from build123d import *

# Parameters (mm, degrees)
SKETCH1_W            = 1017.150431592
SKETCH1_H            = 1007.380411388
BOSS_EXTRUDE1_DEPTH  = 10
SKETCH2_W            = 622.325209365
SKETCH2_H            = 576.276335175
SKETCH2_W_2          = 550.905616221
SKETCH2_H_2          = 495.653174758
BOSS_EXTRUDE2_DEPTH  = 700
BOSS_EXTRUDE3_DEPTH  = 10
SKETCH4_W            = 343.745663019
SKETCH4_H            = 631.457492732
CUT_EXTRUDE1_DEPTH   = 40
SKETCH5_W            = 96.085656893
SKETCH5_H            = 209.087602639
BOSS_EXTRUDE4_DEPTH  = 1
SKETCH6_W            = 75.527574186
SKETCH6_H            = 43.688329808
CUT_EXTRUDE2_DEPTH   = 1
SKETCH7_R            = 20.29708438
SKETCH7_R_2          = 20.231985555
BOSS_EXTRUDE5_DEPTH  = 1
BOSS_EXTRUDE6_DEPTH  = 1
SKETCH9_W            = 27.290112983
SKETCH9_H            = 631.457492732
BOSS_EXTRUDE7_DEPTH  = 170
SKETCH10_W           = 23.826275683
SKETCH10_H           = 630.503372623
BOSS_EXTRUDE8_DEPTH  = 170
SKETCH11_W           = 102.432085561
SKETCH11_H           = 42.683052162
BOSS_EXTRUDE9_DEPTH  = 1
SKETCH12_W           = 89.43349782
SKETCH12_H           = 33.905937228
CUT_EXTRUDE3_DEPTH   = 1
BOSS_EXTRUDE10_DEPTH = 1
BOSS_EXTRUDE11_DEPTH = 1
BOSS_EXTRUDE12_DEPTH = 1
SKETCH16_W           = 75.527574186
SKETCH16_H           = 43.688329808
CUT_EXTRUDE4_DEPTH   = 2
CUT_EXTRUDE5_DEPTH   = 1
SKETCH18_W           = 75.494640665
SKETCH18_H           = 38.009856791
CUT_EXTRUDE6_DEPTH   = 3
BOSS_EXTRUDE14_DEPTH = 2
BOSS_EXTRUDE15_DEPTH = 2


with BuildPart() as part:
    # Sketch1 → Boss-Extrude1 (new body)
    with BuildSketch(Plane(origin=(0, 0, 0), x_dir=(1, 0, 0), z_dir=(0, 1, 0))):
        Rectangle(SKETCH1_W, SKETCH1_H)
    extrude(amount=BOSS_EXTRUDE1_DEPTH)

    # Sketch2 → Boss-Extrude2 (add)
    with BuildSketch(Plane(origin=(0, 10, 0), x_dir=(1, 0, 0), z_dir=(0, 1, 0))):
        with Locations((0.175057265, -25.815388539)):
            Rectangle(SKETCH2_W, SKETCH2_H)
        with Locations((3.438260109, -29.815460152)):
            Rectangle(SKETCH2_W_2, SKETCH2_H_2, mode=Mode.SUBTRACT)
    extrude(amount=BOSS_EXTRUDE2_DEPTH)

    # Sketch3 → Boss-Extrude3 (add)
    with BuildSketch(Plane(origin=(0, 710, 0), x_dir=(1, 0, 0), z_dir=(0, 1, 0))):
        Polygon((-310.987547417, 262.322779049), (311.337661948, 262.322779049), (311.337661948, -314.105065769), (-310.987547417, -313.953556126), align=None)
    extrude(amount=BOSS_EXTRUDE3_DEPTH)

    # Sketch4 → Cut-Extrude1 (cut)
    with BuildSketch(Plane.XY.offset(313.953556126)):
        with Locations((1.971257292, 325.728746366)):
            Rectangle(SKETCH4_W, SKETCH4_H)
    extrude(amount=-CUT_EXTRUDE1_DEPTH, mode=Mode.SUBTRACT)

    # Sketch5 → Boss-Extrude4 (add)
    with BuildSketch(Plane.XY.offset(313.953556126)):
        with Locations((-235.628465158, 369.989290471)):
            Rectangle(SKETCH5_W, SKETCH5_H)
    extrude(amount=BOSS_EXTRUDE4_DEPTH)

    # Sketch6 → Cut-Extrude2 (cut)
    with BuildSketch(Plane.XY.offset(314.953556126)):
        with Locations((-233.410831007, 396.905866965)):
            Rectangle(SKETCH6_W, SKETCH6_H)
    extrude(amount=-CUT_EXTRUDE2_DEPTH, mode=Mode.SUBTRACT)

    # Sketch7 → Boss-Extrude5 (add)
    with BuildSketch(Plane.XY.offset(314.953556126)):
        with Locations((-236.075713016, 343.617219623)):
            Circle(SKETCH7_R)
        with Locations((-236.075713016, 291.501520139)):
            Circle(SKETCH7_R_2)
    extrude(amount=BOSS_EXTRUDE5_DEPTH)

    # Sketch8 → Boss-Extrude6 (add)
    with BuildSketch(Plane.XY.offset(315.953556126)):
        Polygon((-248.100542069, 334.343180385), (-224.116847865, 334.343180385), (-236.108694967, 356.570085863), align=None)
        Polygon((-248.100542069, 300.734143469), (-224.116847865, 300.734143469), (-236.108694967, 278.021129489), align=None)
    extrude(amount=BOSS_EXTRUDE6_DEPTH)

    # Sketch9 → Boss-Extrude7 (add)
    with BuildSketch(Plane(origin=(-169.901574217, 0, 0), x_dir=(0, 0, -1), z_dir=(1, 0, 0))):
        with Locations((-291.287104022, 325.728746366)):
            Rectangle(SKETCH9_W, SKETCH9_H)
    extrude(amount=BOSS_EXTRUDE7_DEPTH)

    # Sketch10 → Boss-Extrude8 (add)
    with BuildSketch(Plane(origin=(0.098425783, 0, 0), x_dir=(0, 0, -1), z_dir=(1, 0, 0))):
        with Locations((-289.555185372, 325.251686312)):
            Rectangle(SKETCH10_W, SKETCH10_H)
    extrude(amount=BOSS_EXTRUDE8_DEPTH)

    # Sketch11 → Boss-Extrude9 (add)
    with BuildSketch(Plane.XY.offset(313.953556126)):
        with Locations((-2.491684156, 672.586316149)):
            Rectangle(SKETCH11_W, SKETCH11_H)
    extrude(amount=BOSS_EXTRUDE9_DEPTH)

    # Sketch12 → Cut-Extrude3 (cut)
    with BuildSketch(Plane.XY.offset(314.953556126)):
        with Locations((-2.82995258, 672.168915251)):
            Rectangle(SKETCH12_W, SKETCH12_H)
    extrude(amount=-CUT_EXTRUDE3_DEPTH, mode=Mode.SUBTRACT)

    # Sketch13 → Boss-Extrude10 (add)
    with BuildSketch(Plane.XY.offset(313.953556126)):
        Polygon((-16.188659158, 682.333537789), (-12.363636267, 682.333537789), (-16.280886962, 666.180161515), (-10.826136902, 666.180161515), (-10.826136902, 671.523280071), (-7.909927509, 671.523280071), (-7.909927509, 666.180161515), (-5.371386842, 666.180161515), (-5.371386842, 662.797245592), (-7.909927509, 662.797245592), (-7.909927509, 659.936990738), (-10.826136902, 659.936990738), (-10.826136902, 662.797245592), (-21.28940391, 662.797245592), align=None)
    extrude(amount=BOSS_EXTRUDE10_DEPTH)

    # Sketch14 → Boss-Extrude11 (add)
    with BuildSketch(Plane.XY.offset(313.953556126)):
        Polygon((8.28251296, 678.526064939), (25.453577984, 678.526064939), (16.868045472, 660.40217423), align=None)
    extrude(amount=BOSS_EXTRUDE11_DEPTH)

    # Sketch15 → Boss-Extrude12 (add)
    with BuildSketch(Plane.XY.offset(313.953556126)):
        Polygon((-253.392365097, 406.408287302), (-253.392365097, 387.565087067), (-258.932297981, 387.565087067), (-258.932297981, 385.030446751), (-244.376138332, 385.030446751), (-244.376138332, 387.568096861), (-249.880180429, 387.568096861), (-249.880180429, 410.563051887), (-259.692933011, 410.252172121), (-259.566620724, 406.408287302), align=None)
    extrude(amount=BOSS_EXTRUDE12_DEPTH)

    # Sketch16 → Cut-Extrude4 (cut)
    with BuildSketch(Plane.XY.offset(313.953556126)):
        with Locations((-233.410831007, 396.905866965)):
            Rectangle(SKETCH16_W, SKETCH16_H)
        Polygon((-258.932297981, 387.565087067), (-253.392365097, 387.565087067), (-253.392365097, 406.408287302), (-259.566620724, 406.408287302), (-259.692933011, 410.252172121), (-249.880180429, 410.563051887), (-249.880180429, 387.568096861), (-244.376138332, 387.568096861), (-244.376138332, 385.030446751), (-258.932297981, 385.030446751), align=None, mode=Mode.SUBTRACT)
        with BuildLine():
            Line((-235.648545177, 385.585769087), (-235.648545177, 408.465773981))
            Line((-235.648545177, 408.465773981), (-231.895053527, 408.465773981))
            Line((-231.895053527, 408.465773981), (-231.895053527, 406.607783771))
            ThreePointArc((-231.895053527, 406.607783771), (-226.013052079, 408.340663022), (-220.604725505, 405.450885314))
            ThreePointArc((-220.604725505, 405.450885314), (-212.450287881, 408.121471894), (-206.512581436, 401.927077024))
            Line((-206.512581436, 401.927077024), (-206.270978925, 385.585769087))
            Line((-206.270978925, 385.585769087), (-208.886279481, 385.585769087))
            Line((-208.886279481, 385.585769087), (-208.886279481, 401.591739947))
            ThreePointArc((-208.886279481, 401.591739947), (-213.544522639, 405.905815865), (-219.282803566, 403.188719557))
            Line((-219.282803566, 403.188719557), (-219.086260967, 397.970062451))
            Line((-219.086260967, 397.970062451), (-218.821188952, 385.585769087))
            Line((-218.821188952, 385.585769087), (-221.983422689, 385.585769087))
            Line((-221.983422689, 385.585769087), (-221.983422689, 403.056833873))
            ThreePointArc((-221.983422689, 403.056833873), (-227.433038153, 405.693579889), (-232.223072214, 401.991376226))
            Line((-232.223072214, 401.991376226), (-232.106265572, 385.585769087))
            Line((-232.106265572, 385.585769087), (-235.648545177, 385.585769087))
        make_face(mode=Mode.SUBTRACT)
    extrude(amount=-CUT_EXTRUDE4_DEPTH, mode=Mode.SUBTRACT)

    # Sketch17 → Cut-Extrude5 (cut)
    with BuildSketch(Plane.XY.offset(311.953556126)):
        Polygon((-271.209439503, 458.857228745), (-195.647043914, 458.857228745), (-195.704078741, 418.44137546), (-271.209439503, 418.44137546), align=None)
    extrude(amount=-CUT_EXTRUDE5_DEPTH, mode=Mode.SUBTRACT)

    # Sketch18 → Cut-Extrude6 (cut)
    with BuildSketch(Plane.XY.offset(314.953556126)):
        with Locations((-233.394364247, 437.754960265)):
            Rectangle(SKETCH18_W, SKETCH18_H)
    extrude(amount=-CUT_EXTRUDE6_DEPTH, mode=Mode.SUBTRACT)

    # Sketch19 → Boss-Extrude14 (add)
    with BuildSketch(Plane.XY.offset(310.953556126)):
        Polygon((-254.312852224, 446.740647117), (-254.312852224, 426.35566573), (-259.396180858, 426.35566573), (-259.396180858, 423.275008449), (-244.678284124, 423.275008449), (-244.678284124, 426.345347073), (-250.728067912, 426.345347073), (-250.728067912, 450.11543046), (-259.396180858, 450.11543046), (-259.396180858, 446.740647117), align=None)
    extrude(amount=BOSS_EXTRUDE14_DEPTH)

    # Sketch20 → Boss-Extrude15 (add)
    with BuildSketch(Plane.XY.offset(310.953556126)):
        with BuildLine():
            Line((-231.738910846, 449.836701393), (-231.738910846, 423.361516406))
            Line((-231.738910846, 423.361516406), (-228.297984767, 423.361516406))
            Line((-228.297984767, 423.361516406), (-228.145561752, 436.327846212))
            ThreePointArc((-228.145561752, 436.327846212), (-216.928259639, 443.252630869), (-228.56606882, 449.444715067))
            Line((-228.56606882, 449.444715067), (-228.61564163, 450.293665645))
            Line((-228.61564163, 450.293665645), (-231.738910846, 450.293665645))
            Line((-231.738910846, 450.293665645), (-231.738910846, 449.836701393))
        make_face()
        with BuildLine():
            Line((-228.56606882, 446.492870427), (-228.297984767, 439.236609845))
            ThreePointArc((-228.297984767, 439.236609845), (-219.191503534, 443.206133185), (-228.56606882, 446.492870427))
        make_face(mode=Mode.SUBTRACT)
    extrude(amount=BOSS_EXTRUDE15_DEPTH)


solid = part.part
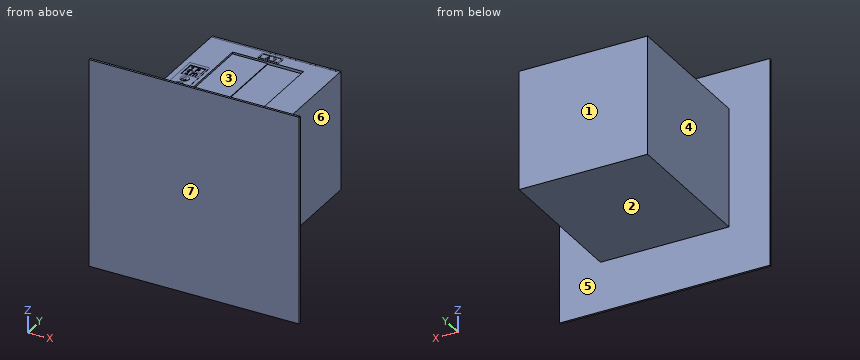
For this review, take the finished solid that the model builds, in its own axes (mm). Face numbers are marked on the shaded views. A direction names the side the tool comes from. Coordinates: 2 decimals unless noted, no trailing zeros. Loops run counter-clockwise (first coordinate to the right, second up) from the corner with the lowest first, then second, coordinate; pieces in that order, holes last. Notation, with made-up numbers: (-40, 63) - (-16, 63) arc R31 ccw to (-16, 88) - close; hole circle Ø1 at (84.5, 69). An arc over 180 degrees is marked (long way). Return JSON: item names as keys, results as strings.
Item 1: Mouldability with a two-part tool opening along X and no side actions: class the marked faces 5, 6 and 7 as pulls with the +X half, pulls with the -X half, needs draft (parallel to the pull), parting line crosses it, or undercut.
Determined:
{"face 5": "undercut", "face 6": "pulls with the +X half", "face 7": "needs draft"}
Item 2: Take a section at B-B (y = 230.5). Give the boundary of the cut face in (x, z), then the cut area to 3 significant figures.
Determined:
{"outline": "(-310.99, -262.32) - (311.34, -262.32) - (311.34, 313.95) - (173.84, 313.95) - (173.84, 277.64) - (278.89, 277.64) - (278.89, -218.01) - (-272.01, -218.01) - (-272.01, 277.64) - (170.1, 277.64) - (170.1, 301.47) - (0.1, 301.47) - (0.1, 304.93) - (-169.9, 304.93) - (-169.9, 313.95) - (-310.99, 313.95) - close", "area": "81,800 mm2"}
Item 3: Take a section at C-C (z = -242.5). Give the boundary of the cut face in (x, y), then the cut area to 3 significant figures.
Determined:
{"outline": "(-508.58, 0) - (508.58, 0) - (508.58, 10) - (311.34, 10) - (311.34, 720) - (-310.99, 720) - (-310.99, 10) - (-508.58, 10) - close", "area": "452,000 mm2"}
Item 4: Take a section at A-A (z = 70.5). Give the boundary of the cut face in (x, y).
Determined:
{"outline": "(-508.58, 0) - (508.58, 0) - (508.58, 10) - (311.34, 10) - (311.34, 720) - (-310.99, 720) - (-310.99, 10) - (-508.58, 10) - close; hole (-272.01, 10) - (278.89, 10) - (278.89, 710) - (-272.01, 710) - close"}
Item 5: Insertion check: pin 1 (1.5 mm diameter, centred on y = 387, z = 314, fed in from +X); pin 2 (6 mm diameter, centred on x = -30, z = -281, fed in from +Y); pin 3 (0.5 mm diameter, centred on x = 19, z = 314.5, fed in from +Y). Each pin has a flat end and moves straight along its axis. Give the tip position at first contact, or say it passes through.
Determined:
{"pin 1": "stops at x = 311.34", "pin 2": "stops at y = 10", "pin 3": "stops at y = 693.93"}
Item 6: For line 1 (Z direction, x = 142, y = 681); line 2 (X direction, y = 534, z = -174); line 3 (Y direction, x = -224.5, z = -158.5), list the stretches that pass through material, from the lowest coordinate up.
Determined:
{"line 1": "z = -262.32 to -218.01, 277.64 to 313.95", "line 2": "x = -310.99 to -272.01, 278.89 to 311.34", "line 3": "y = 0 to 10, 710 to 720"}
Item 7: Take a section at D-D (x = -84.5). Give the boundary of the cut face in (y, z).
Determined:
{"outline": "(0, -503.69) - (10, -503.69) - (10, -262.32) - (720, -262.32) - (720, 314.01) - (710, 314.01) - (710, 313.95) - (641.46, 313.95) - (641.46, 304.93) - (10, 304.93) - (10, 503.69) - (0, 503.69) - close; hole (10, -218.01) - (710, -218.01) - (710, 277.64) - (10, 277.64) - close"}
Item 8: For the marked faces 1, 2, 3 and 4, list the 3-axis set-ups (+Z, -Z, +X, -X, +Y, -Y) from which the entire face can be reached by the end or side of a thin tool; tool diameter is ignored.
Determined:
{"face 1": "+Z, -Z, +X, -X, +Y", "face 2": "-Z, +X, -X, +Y", "face 3": "+Z", "face 4": "+Z, -Z, -X, +Y"}
